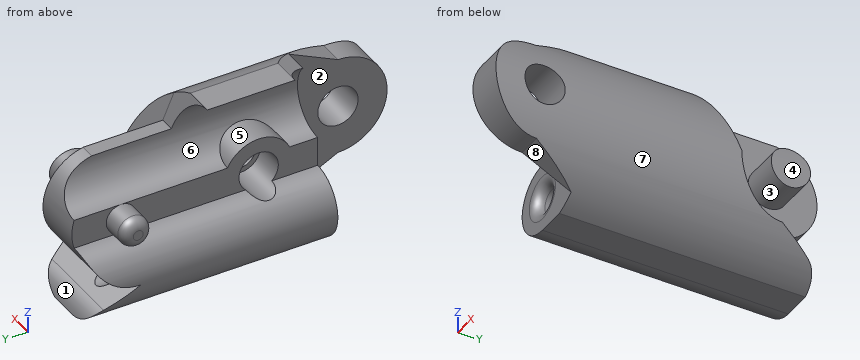
from build123d import *

# Parameters (mm, degrees)
BOSS_EXTRUDE1_DEPTH = 35
SKETCH2_R           = 1.27
CUT_EXTRUDE1_DEPTH  = 35
CUT_EXTRUDE2_REACH  = 41.937
SKETCH3_W           = 10
SKETCH3_H           = 10
SKETCH4_R           = 2.049999964
CUT_EXTRUDE3_DEPTH  = 17.5
CUT_EXTRUDE5_START  = -7.95804
SKETCH6_R           = 2
CUT_EXTRUDE5_DEPTH  = 9.6
FILLET3_R           = 1
CUT_EXTRUDE6_START  = 8.64596
SKETCH6_3_R         = 2
CUT_EXTRUDE6_DEPTH  = 6.604
CUT_EXTRUDE7_START  = -14.986
CUT_EXTRUDE7_DEPTH  = 14.986
CUT_EXTRUDE8_DEPTH  = 31.496
SKETCH9_R           = 1.5
CUT_EXTRUDE9_DEPTH  = 8.382
SKETCH11_R          = 2
CUT_EXTRUDE10_DEPTH = 3.1
BOSS_EXTRUDE2_DEPTH = 3.862
SKETCH13_R          = 1.5
BOSS_EXTRUDE4_DEPTH = 3
FILLET5_R           = 1


with BuildPart() as part:
    # Sketch1 → Boss-Extrude1 (new body)
    with BuildSketch(Plane(origin=(0, 0, 0), x_dir=(1, 0, 0), z_dir=(0, 1, 0))):
        with BuildLine():
            Line((-2.958039892, 8.5), (2.958039892, 8.5))
            ThreePointArc((2.958039892, 8.5), (9, 0), (2.958039892, -8.5))
            Line((2.958039892, -8.5), (-2.958039892, -8.5))
            ThreePointArc((-2.958039892, -8.5), (-9, 0), (-2.958039892, 8.5))
        make_face()
    extrude(amount=BOSS_EXTRUDE1_DEPTH)

    # Sketch2 → Cut-Extrude1 (cut)
    with BuildSketch(Plane.XZ):
        with Locations(Location((0, -5, 0), (0, 0, 270))):
            Circle(SKETCH2_R)
        with Locations(Location((0, 5, 0), (0, 0, 270))):
            Circle(SKETCH2_R)
    extrude(amount=-CUT_EXTRUDE1_DEPTH, mode=Mode.SUBTRACT)

    # Cut-Extrude2: up to this face of the body (flat: up to its plane)
    cut_extrude2_end = Plane(part.part.faces().sort_by_distance((0, 17.5, 8.5))[0])
    # Sketch3 → Cut-Extrude2 (cut, up to the picked face)
    with BuildSketch(Plane(origin=(0, 0, -8.5), x_dir=(-1, 0, 0), z_dir=(0, 0, -1)), mode=Mode.PRIVATE) as cut_extrude2_sk1:
        with Locations((0, 5)):
            Rectangle(SKETCH3_W, SKETCH3_H)
    cut_extrude2_tool1 = split(extrude(cut_extrude2_sk1.sketch, amount=-CUT_EXTRUDE2_REACH, mode=Mode.PRIVATE), bisect_by=cut_extrude2_end, keep=Keep.BOTH, mode=Mode.PRIVATE)
    add(cut_extrude2_tool1.solids().sort_by(Axis((0, 5, -8.5), (0, 0, 1)))[0], mode=Mode.SUBTRACT)

    # Sketch4 → Cut-Extrude3 (cut, symmetric)
    with BuildSketch(Plane.ZY.offset(-5)):
        with Locations(Location((0, 5, 0), (0, 0, 270))):
            Circle(SKETCH4_R)
        with BuildLine():
            Line((-7.483314774, 10), (-5, 5))
            ThreePointArc((-5, 5), (0, 0), (5, 5))
            Line((5, 5), (8.5, 12.308552788))
            Line((8.5, 12.308552788), (9.857943437, -1.822240199))
            Line((9.857943437, -1.822240199), (-9.857943437, -1.822240199))
            Line((-9.857943437, -1.822240199), (-7.483314774, 10))
        make_face()
    extrude(amount=CUT_EXTRUDE3_DEPTH, both=True, mode=Mode.SUBTRACT)

    # Sketch6 → Cut-Extrude5 (cut)
    with BuildSketch(Plane.ZY.offset(2.958039892).offset(CUT_EXTRUDE5_START)):
        with BuildLine():
            Line((8.5, 21.219917379), (0, 25))
            ThreePointArc((0, 25), (-3.535533906, 26.464466094), (-5, 30))
            Line((-5, 30), (-6.755867779, 33.535330675))
            ThreePointArc((-6.755867779, 33.535330675), (-7.475170692, 34.449576169), (-8.5, 35))
            Line((-8.5, 35), (17.803004008, 42.886049022))
            Line((17.803004008, 42.886049022), (8.5, 21.219917379))
        make_face()
        with Locations((0, 30)):
            Circle(SKETCH6_R, mode=Mode.SUBTRACT)
    extrude(amount=-CUT_EXTRUDE5_DEPTH, mode=Mode.SUBTRACT)

    # Fillet3
    fillet3_edges = [part.edges().sort_by_distance(p)[0] for p in [
        (0, 10, -3.73),
        (0, 10, 6.27),
    ]]
    fillet(fillet3_edges, radius=FILLET3_R)

    # Sketch6<3> → Cut-Extrude6 (cut)
    with BuildSketch(Plane.ZY.offset(2.958039892).offset(CUT_EXTRUDE6_START)):
        with BuildLine():
            Line((8.5, 21.219917379), (0, 25))
            ThreePointArc((0, 25), (-3.535533906, 26.464466094), (-5, 30))
            Line((-5, 30), (-6.755867779, 33.535330675))
            ThreePointArc((-6.755867779, 33.535330675), (-7.475170692, 34.449576169), (-8.5, 35))
            Line((-8.5, 35), (17.803004008, 42.886049022))
            Line((17.803004008, 42.886049022), (8.5, 21.219917379))
        make_face()
        with Locations((0, 30)):
            Circle(SKETCH6_3_R, mode=Mode.SUBTRACT)
    extrude(amount=-CUT_EXTRUDE6_DEPTH, mode=Mode.SUBTRACT)

    # Sketch7 → Cut-Extrude7 (cut)
    with BuildSketch(Plane(origin=(5, 0, 0), x_dir=(0, 0, -1), z_dir=(1, 0, 0)).offset(CUT_EXTRUDE7_START)):
        with BuildLine():
            Line((5, 30), (6.755867779, 33.535330675))
            ThreePointArc((6.755867779, 33.535330675), (7.475170692, 34.449576169), (8.5, 35))
            Line((8.5, 35), (-8.341946035, 47.536710192))
            Line((-8.341946035, 47.536710192), (-13.168237897, 33.528506419))
            Line((-13.168237897, 33.528506419), (-10.04678731, 20.532036929))
            Line((-10.04678731, 20.532036929), (-4.915473018, 22.814012455))
            Line((-4.915473018, 22.814012455), (-4.915473018, 30.915491676))
            ThreePointArc((-4.915473018, 30.915491676), (0.459692783, 34.97882341), (5, 30))
        make_face()
    extrude(amount=CUT_EXTRUDE7_DEPTH, mode=Mode.SUBTRACT)

    # Sketch8 → Cut-Extrude8 (cut, symmetric)
    with BuildSketch(Plane.XZ.offset(-10)):
        with BuildLine():
            Line((0, 1.5), (0, -1.5))
            ThreePointArc((0, -1.5), (-3.5, -5), (0, -8.5))
            Line((0, -8.5), (-4.790142834, -16.013604782))
            Line((-4.790142834, -16.013604782), (-17.855559142, -9.717705198))
            Line((-17.855559142, -9.717705198), (-4.790142834, 15.219000931))
            Line((-4.790142834, 15.219000931), (0, 8.5))
            ThreePointArc((0, 8.5), (3.5, 5), (0, 1.5))
        make_face()
    extrude(amount=CUT_EXTRUDE8_DEPTH, both=True, mode=Mode.SUBTRACT)

    # Sketch9 → Cut-Extrude9 (cut)
    with BuildSketch(Plane.ZY):
        with Locations((0, 16)):
            Circle(SKETCH9_R)
    extrude(amount=-CUT_EXTRUDE9_DEPTH, mode=Mode.SUBTRACT)

    # Sketch11 → Cut-Extrude10 (cut, symmetric)
    with BuildSketch(Plane.ZY):
        with Locations((0, 16)):
            Circle(SKETCH11_R)
    extrude(amount=CUT_EXTRUDE10_DEPTH, both=True, mode=Mode.SUBTRACT)

    # Sketch12 → Boss-Extrude2 (add)
    with BuildSketch(Plane.ZY):
        with BuildLine():
            Line((0, 18), (0, 19.5))
            ThreePointArc((0, 19.5), (3.5, 16), (0, 12.5))
            Line((0, 12.5), (0, 14))
            ThreePointArc((0, 14), (2, 16), (0, 18))
        make_face()
    extrude(amount=-BOSS_EXTRUDE2_DEPTH)

    # Sketch13 → Boss-Extrude4 (add)
    with BuildSketch(Plane.ZY):
        with Locations((0, 30)):
            Circle(SKETCH13_R)
    extrude(amount=BOSS_EXTRUDE4_DEPTH)

    # Fillet5
    fillet5_edges = [part.edges().sort_by_distance(p)[0] for p in [
        (-3, 30, -1.5),
    ]]
    fillet(fillet5_edges, radius=FILLET5_R)


solid = part.part
Verification items for the finished model (mm, model axes). Face numbers are marked on the shaded views. A direction names the side the tool comes from. Give positions to 0.01 mm unless a question says otherwise; leave off trailing zeros. Order: outer loops, then holes, each group sorted by start corner. A loop starts at its lowest first (then second) coordinate and runs counter-clockwise, first axis right, second up. Notation, with made-up numbers: M 51.5,88.25 L 59.5,88.25 A17 ccw 59.5,109.25 Z; hole C 59.25,-16 d4. An arc over 180 degrees is marked long. Answer as a JSON object with one key per item and string values. Group by question number.
1) Cross-section at A-A (y = 18.5). Enter the section's corners in (x, z).
2) Depth check by flat-ended pin: pin 1 Ø2 at (x, z) = (3.5, 3.5) entering from +Y; pin 2 Ø2.5 at (y, z) = (16, 0) entering from -X; pin 3 Ø1.5 at (y, z) = (21, 0.5) entering from -X; pin 4 Ø6 at (x, y) = (4, 20.5) entering from -Z. Enter the tip coordinate at first touch or a pass-through.
3) Scan lines: line 1 along Y through (x, z) = (6.45, 0); line 2 along Z through (x, y) = (7.2, 5); line 3 along Y through (x, z) = (0.8, 0). Record each from-to range of solid material in increasing order. Write a range as [from, to].
4) Cross-section at C-C (z = 5.75). Enter the section's corners in (x, y), then the cut area to 3 significant figures.
5) Access from +Z, -Z, +X, -X, +Y, -Y to the whole of each face (thin tool, end or side, straight path). Record for the marked faces 1, 2, 3, 4 and 5.
6) Mould release check, pull along Z, two halves, no side actions. Record for the marked faces 6, 7 and 8: released by +Z, released by -Z, zero draft, split by the parting line, or undercut.
7) Cross-section at D-D (y = 25.5). Enter the section's corners in (x, z).
8) Cross-section at B-B (x = 0.75). Give the number of separate pieces and of enclosed holes in the cut face, then the cut area to 3 significant figures.
Result sheet:
{
 "1": {"outline": "M 0,-8.5 L 2.96,-8.5 A9 ccw 2.96,8.5 L 0,8.5 A3.5 cw 2.4,2.45 L 0,2.45 L 0,-1.5 A3.5 ccw Z; hole C 0,-5 d2.54"},
 "2": {"pin 1": "stops at y = 34.33", "pin 2": "stops at x = 8.38", "pin 3": "stops at x = 0", "pin 4": "stops at z = -8.5"},
 "3": {"line 1": "y = [0, 2.95], [7.05, 14.5], [17.5, 25], [28, 32]", "line 2": "z = [-5, -2.05], [2.05, 5]", "line 3": "y = [10, 14], [18, 35]"},
 "4": {"outline": "M 3.42,10 L 5,10 L 5,6.57 L 6.92,6.57 L 6.92,22.44 L 3.42,22.44 Z", "area": "50.2 mm2"},
 "5": {"face 1": "+X, -X, +Y", "face 2": "+Z, -Z, -X, -Y", "face 3": "+X", "face 4": "+X, +Y, -Y", "face 5": "-X"},
 "6": {"face 6": "undercut", "face 7": "split by the parting line", "face 8": "released by -Z"},
 "7": {"outline": "M 0,-8.5 L 2.96,-8.5 A9 ccw 8.73,-2.18 L 5,-2.18 L 5,4.92 L 3.5,4.92 A3.5 cw 0,1.5 L 0,-1.5 A3.5 ccw Z; hole C 0,-5 d2.54"},
 "8": {"separate pieces": "3", "enclosed holes": "1", "area": "192 mm2"}
}
